Autodesk Inventor part; units mm, degrees
ref_plane "YZ Plane" through (0, 0, 0) normal (1, 0, 0) x (0, 1, 0)
ref_plane "XZ Plane" through (0, 0, 0) normal (0, 1, 0) x (-1, 0, 0)
ref_plane "XY Plane" through (0, 0, 0) normal (0, 0, 1) x (1, 0, 0)
sketch "Sketch1" plane through (0, 0, 0) normal (0, 0, 1) x (1, 0, 0)
  circle A0 centre (0, 0) radius 3.175
  dimension "d0" = 6.35
extrude "Extrusion1" add sketch "Sketch1" along normal mid plane 15.875
sketch "Sketch2" plane through (0, 0, 7.9375) normal (0, 0, 1) x (1, 0, 0)
  circle A0 centre (0, 0) radius 3.175
hole "Hole1" at (0, 0, 7.9375) direction (0, 0, -1) diameter 4.9276 end through all
chamfer "Chamfer1" distance 0.254 angle 45 2 edges at (-3.175, 0, 7.9375) (-3.175, 0, -7.9375)
properties part number "Elevator Cascade Pulley Bearing Spacer" material "Aluminum"
Design review of the part built by this model. Coordinates are the model's own, in mm. Give positions to 0.01 mm unless a question says otherwise; leave off trailing zeros. Order: outer loops, then holes, each group sorted by start corner. A loop starts at its lowest first (then second) coordinate and runs counter-clockwise, first axis right, second up. Notation, with made-up numbers: (-25.5, 6) - (-20.5, 6) arc R31 cw to (-20.5, 44) - close; hole circle Ø6 at (34, 71.5). An arc over 180 degrees is marked (long way). Use a Markdown table: item, result. Add a question column.
(1) Add section C-C on z = -4.5. Give the boundary of the cut face in (x, y) (3 decimals), then the cut area to 3 significant figures.
(2) Mouldability with a two-part tool opening along Y and no side actions: class faces 1 (the face through (-0.69, 3.1, -0.11)), 2 (the face through (-0.11, 2.46, -0.11)) as +Y half, -Y half, draft (parallel to the pull), parting line (faces both ways), or undercut.
(3) Wall thickness on probe 1 along Y at (x, z) = (0, 2.75) (3 decimals); probe 2 along X at (y, z) = (0.5, -6.5); probe 3 along X at (y, z) = (2.25, 4.5): over which ranges is each line inside the solid? List them lowest first. Write a range as [from, to].
Report:
| question | item | result |
|---|---|---|
| 1 | outline | circle Ø6.35 at (0, 0); hole circle Ø4.928 at (0, 0) |
| 1 | area | 12.6 mm² |
| 2 | face 1 | parting line |
| 2 | face 2 | undercut |
| 3 | probe 1 | y = [-3.175, -2.464], [2.464, 3.175] |
| 3 | probe 2 | x = [-3.14, -2.41], [2.41, 3.14] |
| 3 | probe 3 | x = [-2.24, -1], [1, 2.24] |
